Could you check a few things on this model? Use its own coordinates, in mm. A direction names the side the tool comes from. Coordinates: 2 decimals unless noted, no trailing zeros. Loops run counter-clockwise (first coordinate to the right, second up) from the corner with the lowest first, then second, coordinate; pieces in that order, holes last.
from build123d import *

# Parameters (mm, degrees)
F0_W      = 32
F0_H      = 32
F1_DEPTH  = 8
F2_W      = 10
F2_H      = 20
F2_H_2    = 5.5
F3_DEPTH  = 10
F5_DEPTH  = 6
F6_R      = 3
F7_DEPTH  = 25
F8_R      = 3
F9_DEPTH  = 25
F10_R     = 3
F11_DEPTH = 32.001
F12_R     = 4.99999
F13_R     = 4.99999
F14_R     = 5


# Not quite as in the source:
# - a fillet or chamfer is up to 0.001 mm smaller than in the source, because OpenCascade refuses the exact size


with BuildPart() as f1:
    # F0 (on Front) → F1 (new body)
    with BuildSketch(Plane.XZ):
        Rectangle(F0_W, F0_H)
    extrude(amount=F1_DEPTH)

    # F2 (on face) → F3 (join)
    with BuildSketch(Plane.XZ.offset(8)):
        with Locations((-11, 0)):
            Rectangle(F2_W, F2_H)
        with Locations((11, -13.25)):
            Rectangle(F2_W, F2_H_2)
        with Locations((11, 13.25)):
            Rectangle(F2_W, F2_H_2)
    extrude(amount=F3_DEPTH)

    # F4 (on face) → F5 (cut)
    with BuildSketch(Plane.XZ.offset(8)):
        Polygon((6, -3.4641016151), (6, 3.4641016151), (0, 6.9282032303), (-6, 3.4641016151), (-6, -3.4641016151), (0, -6.9282032303), align=None)
    extrude(amount=-F5_DEPTH, mode=Mode.SUBTRACT)

    # F6 (on face) → F7 (cut)
    with BuildSketch(Plane(origin=(0, 0, 0), x_dir=(-1, 0, 0), z_dir=(0, 1, 0))):
        Circle(F6_R)
    extrude(amount=-F7_DEPTH, mode=Mode.SUBTRACT)

    # F8 (on face) → F9 (cut)
    with BuildSketch(Plane(origin=(0, 0, -10), x_dir=(1, 0, 0), z_dir=(0, 0, -1))):
        with Locations((-11, 13)):
            Circle(F8_R)
    extrude(amount=-F9_DEPTH, mode=Mode.SUBTRACT)

    # F10 (on face) → F11 (cut, through all)
    with BuildSketch(Plane(origin=(0, 0, -16), x_dir=(1, 0, 0), z_dir=(0, 0, -1))):
        with Locations((11, 13)):
            Circle(F10_R)
    extrude(amount=-F11_DEPTH, mode=Mode.SUBTRACT)

    # F12 (radius 5 in the source; OpenCascade refuses exactly that, so slightly less here)
    f12_edges = [f1.edges().sort_by_distance(p)[0] for p in [
        (6, -18, 13.25),
        (16, -18, 13.25),
        (16, -18, -13.25),
        (6, -18, -13.25),
    ]]
    fillet(f12_edges, radius=F12_R)

    # F13 (radius 5 in the source; OpenCascade refuses exactly that, so slightly less here)
    f13_edges = [f1.edges().sort_by_distance(p)[0] for p in [
        (-6, -18, 0),
        (-16, -18, 0),
    ]]
    fillet(f13_edges, radius=F13_R)

    # F14
    f14_edges = [f1.edges().sort_by_distance(p)[0] for p in [
        (16, -8, 0),
    ]]
    fillet(f14_edges, radius=F14_R)


solid = f1.part
(1) Imagine slicing it at C-C, the plane x = 1. Write out the boundary of the cut face in (y, z).
Answers:
outline: (-8, -16) - (0, -16) - (0, -2.83) - (-2, -2.83) - (-2, -6.35) - (-8, -6.35) - close; (-8, 6.35) - (-2, 6.35) - (-2, 2.83) - (0, 2.83) - (0, 16) - (-8, 16) - close
(2) I need wall thicknesses on probe 1 along X at (y, z) = (-13, -12.95); probe 2 along X at (y, z) = (-13, -4.5); probe 3 along Y at (x, z) = (-11, -5.5). Which ranges of each line are inside material? Lowest first, please.
Answers:
probe 1: x = 6 to 8, 14 to 16
probe 2: x = -16 to -14, -8 to -6
probe 3: y = -18 to -16, -10 to 0
(3) Imagine slicing it at A-A, the plane z = 0. State how many separate pieces and enclosed holes the cut face has, and give its area (3 significant figures).
Answers:
separate pieces: 2
enclosed holes: 1
area: 228 mm2
(4) Which directions (+Z, -Z, +X, -X, +Y, -Y) give clear straight access to the entire face, cutting with the end or side of a thin tool? Please do faces 4 (the face through (14, -7, 0)), 5 (the face through (16, -2, -4)), 6 (the face through (8.6, -11.2, 13.2)), 7 (the face through (-3, -8, -7)), 8 (the face through (-8.8, -10.7, 10)).
Answers:
face 4: +X, -Y
face 5: +Z, -Z, +X, +Y, -Y
face 6: +Z, -Z
face 7: -Y
face 8: +Z, +X, -X, -Y
(5) We'd pull the mould along X, two halves only. Please class faces 1 (the face through (6, -10, -13)), 2 (the face through (-13.4, -11.2, -0.1)), 3 (the face through (15, -16, 13)): +X half, -X half, draft (parallel to the pull), parting line (faces both ways), or undercut.
Answers:
face 1: -X half
face 2: undercut
face 3: +X half
(6) Imagine slicing it at B-B, the plane y = -6.5. Write out the boundary of the cut face in (x, z).
Answers:
outline: (-16, -16) - (16, -16) - (16, -10.5) - (14.57, -10.5) - (14.57, 10.5) - (16, 10.5) - (16, 16) - (-16, 16) - close; hole (-6, -3.46) - (0, -6.93) - (6, -3.46) - (6, 3.46) - (0, 6.93) - (-6, 3.46) - close
(7) For pin 1 (5.5 mm diameter, centred on y = -11, z = 13, fed in from -X); pin 2 (9.5 mm diameter, centred on x = -11, y = -13, fed in from -Z); pin 3 (5.5 mm diameter, centred on y = -10.5, z = -14, fed in from -X); pin 4 (8 mm diameter, centred on x = 0, z = 0, fed in from -Y), each with a flat end and sliding along its axis, tell me the tip position at first contact or that it passes through.
Answers:
pin 1: stops at x = 6
pin 2: stops at z = -10
pin 3: stops at x = -16
pin 4: stops at y = -2
